Work out the finished part from the listing and answer in its coordinate system (mm). A direction names the side the tool comes from. Give positions to 0.01 mm unless a question says otherwise; leave off trailing zeros. Order: outer loops, then holes, each group sorted by start corner. A loop starts at its lowest first (then second) coordinate and runs counter-clockwise, first axis right, second up.
```python
from build123d import *

# Parameters (mm, degrees)
SKETCH1_W             = 10.16
SKETCH1_H             = 41.91
BOSS_EXTRUDE1_DEPTH   = 13.97
SKETCH2_W             = 10.16
SKETCH2_H             = 27.178
CUT_EXTRUDE1_DEPTH    = 9.144
F_3_0MM_DOWEL_HOLE1_D = 3


with BuildPart() as part:
    # Sketch1 → Boss-Extrude1 (new body)
    with BuildSketch(Plane.XY):
        with Locations((5.08, 20.955)):
            Rectangle(SKETCH1_W, SKETCH1_H)
    extrude(amount=BOSS_EXTRUDE1_DEPTH)

    # Sketch2 → Cut-Extrude1 (cut)
    with BuildSketch(Plane.XY.offset(13.97)):
        with Locations((5.08, 20.955)):
            Rectangle(SKETCH2_W, SKETCH2_H)
    extrude(amount=-CUT_EXTRUDE1_DEPTH, mode=Mode.SUBTRACT)

    # Ø3.0mm Dowel Hole1 (through all)
    with Locations(Plane.XY.offset(13.97)):
        with Locations((5.08, 3.683), (5.08, 38.227)):
            Hole(F_3_0MM_DOWEL_HOLE1_D / 2)


solid = part.part
```
1. Straight lines are drawn through the part: probe 1 along Y at (x, z) = (5.08, 4.25); probe 2 along Y at (x, z) = (5.08, 10.25); probe 3 along Y at (x, z) = (7.5, 5). For each, find the intervals that lie inside material, in ascending order.
Findings below:
probe 1: y = 0 to 2.18, 5.18 to 36.73, 39.73 to 41.91
probe 2: y = 0 to 2.18, 5.18 to 7.37, 34.54 to 36.73, 39.73 to 41.91
probe 3: y = 0 to 7.37, 34.54 to 41.91
2. The part is cut by section C-C (x = 3). Write down the section's boundary in (y, z).
Findings below:
outline: (0, 0) - (41.91, 0) - (41.91, 13.97) - (34.54, 13.97) - (34.54, 4.83) - (7.37, 4.83) - (7.37, 13.97) - (0, 13.97) - close
3. The part is cut by section B-B (z = 13.25). Write down the section's boundary in (x, y), then the cut area to 3 significant figures.
Findings below:
outline: (0, 0) - (10.16, 0) - (10.16, 7.37) - (0, 7.37) - close; (0, 34.54) - (10.16, 34.54) - (10.16, 41.91) - (0, 41.91) - close; hole circle Ø3 at (5.08, 3.68); hole circle Ø3 at (5.08, 38.23)
area: 136 mm2
4. The part is cut by section A-A (x = 5.08). Write down the section's boundary in (y, z).
Findings below:
outline: (0, 0) - (2.18, 0) - (2.18, 13.97) - (0, 13.97) - close; (5.18, 0) - (36.73, 0) - (36.73, 13.97) - (34.54, 13.97) - (34.54, 4.83) - (7.37, 4.83) - (7.37, 13.97) - (5.18, 13.97) - close; (39.73, 0) - (41.91, 0) - (41.91, 13.97) - (39.73, 13.97) - close
5. The mould has two halves that part along X. Classify faces 1 (the face through (0, 21, 4)), 2 (the face through (5, 40, 13.97)), 3 (the face through (10.16, 21, 4)), 4 (the face through (6.186, 4.697, 6.887)): pulls with the +X half, pulls with the -X half, needs draft (parallel to the pull), parting line crosses it, or undercut.
Findings below:
face 1: pulls with the -X half
face 2: needs draft
face 3: pulls with the +X half
face 4: undercut
6. The part is cut by section D-D (y = 3). Write down the section's boundary in (x, z), then the cut area to 3 significant figures.
Findings below:
outline: (0, 0) - (3.74, 0) - (3.74, 13.97) - (0, 13.97) - close; (6.42, 0) - (10.16, 0) - (10.16, 13.97) - (6.42, 13.97) - close
area: 105 mm2
7. Which of the six approach directions +Z, -Z, +X, -X, +Y, -Y give full straight-line access (tool end or side, diameter ignored) to faces 5 (the face through (5.405, 36.763, 6.887)), 6 (the face through (5, 34.544, 9))?
Findings below:
face 5: +Z, -Z
face 6: +Z, +X, -X
8. Given P1, Ø4, axis at x = 5, z = 5.5, coming from the -Y side; P2, Ø2.5, axis at x = 5.08, y = 3.683, coming from the +Z side; P3, Ø2, axis at x = 8.5, y = 16, coming from the +Z side, each flat-ended and moving along its own axis, determine where each tip first touches the part or whether it passes through.
Findings below:
P1: stops at y = 0
P2: passes through
P3: stops at z = 4.83
